from build123d import *

# Parameters (mm, degrees)
SKETCH1_W           = 50.8
SKETCH1_H           = 76.2
BOSS_EXTRUDE1_DEPTH = 1.6002
CUT_EXTRUDE1_REACH  = 47.818
SKETCH2_R           = 1.5875


with BuildPart() as part:
    # Sketch1 → Boss-Extrude1 (new body)
    with BuildSketch(Plane.XY):
        Rectangle(SKETCH1_W, SKETCH1_H)
    extrude(amount=BOSS_EXTRUDE1_DEPTH)

    # Sketch2 → Cut-Extrude1 (cut, up to next)
    with BuildSketch(Plane.XY.offset(1.6002), mode=Mode.PRIVATE) as cut_extrude1_sk1:
        with Locations((-21.59, 34.29)):
            Circle(SKETCH2_R)
    cut_extrude1_tool1 = extrude(cut_extrude1_sk1.sketch, amount=-CUT_EXTRUDE1_REACH, mode=Mode.PRIVATE) & part.part
    # Sketch2 → Cut-Extrude1 (cut, up to next)
    with BuildSketch(Plane.XY.offset(1.6002), mode=Mode.PRIVATE) as cut_extrude1_sk2:
        with Locations((21.59, 34.29)):
            Circle(SKETCH2_R)
    cut_extrude1_tool2 = extrude(cut_extrude1_sk2.sketch, amount=-CUT_EXTRUDE1_REACH, mode=Mode.PRIVATE) & part.part
    # Sketch2 → Cut-Extrude1 (cut, up to next)
    with BuildSketch(Plane.XY.offset(1.6002), mode=Mode.PRIVATE) as cut_extrude1_sk3:
        with Locations((21.59, -34.29)):
            Circle(SKETCH2_R)
    cut_extrude1_tool3 = extrude(cut_extrude1_sk3.sketch, amount=-CUT_EXTRUDE1_REACH, mode=Mode.PRIVATE) & part.part
    # Sketch2 → Cut-Extrude1 (cut, up to next)
    with BuildSketch(Plane.XY.offset(1.6002), mode=Mode.PRIVATE) as cut_extrude1_sk4:
        with Locations((-21.59, -34.29)):
            Circle(SKETCH2_R)
    cut_extrude1_tool4 = extrude(cut_extrude1_sk4.sketch, amount=-CUT_EXTRUDE1_REACH, mode=Mode.PRIVATE) & part.part
    add(cut_extrude1_tool1.solids().sort_by_distance((-21.59, 34.29, 1.6002))[0], mode=Mode.SUBTRACT)
    add(cut_extrude1_tool2.solids().sort_by_distance((21.59, 34.29, 1.6002))[0], mode=Mode.SUBTRACT)
    add(cut_extrude1_tool3.solids().sort_by_distance((21.59, -34.29, 1.6002))[0], mode=Mode.SUBTRACT)
    add(cut_extrude1_tool4.solids().sort_by_distance((-21.59, -34.29, 1.6002))[0], mode=Mode.SUBTRACT)


solid = part.part
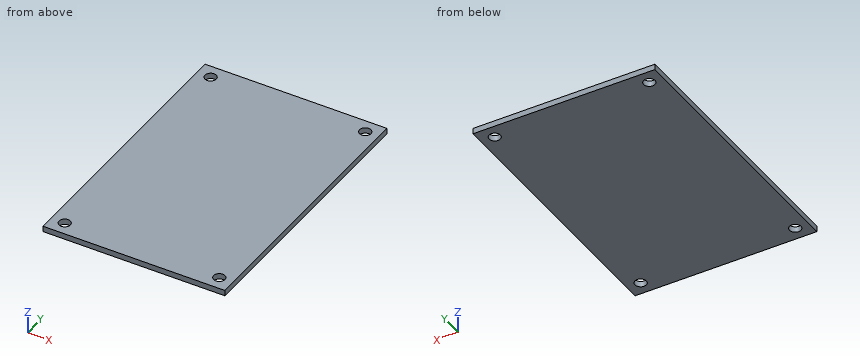
Input: part model. Units: mm. Frame: model coordinates. Coordinates: 2 decimals unless noted, no trailing zeros. Write each loop counter-clockwise with the first axis right and the second up, starting at its lowest first coordinate (ties: lowest second). Pieces come first, ordered by that corner, then holes. Notation, with made-up numbers: M 39,41 L 62,41 A16 cw 62,47 Z; hole C 46.25,47.5 d9. An arc over 180 degrees is marked long. Answer as a JSON object with one key per item and string values. Group by question number.
(1) Section B-B on x = 21.59. Output: boundary loops of the cut face in (y, z), plus the area to 3 significant figures.
(2) Ray query, line 1 along Y through (x, z) = (21.59, 1.2); line 2 along Y through (x, z) = (22, 1.2). Return the intervals inside material, ascending. Write a range as [from, to].
(3) Section A-A on y = 34.29. Output: boundary loops of the cut face in (x, z), plus the area to 3 significant figures.
Result set:
{
 "1": {"outline": "M -38.1,0 L -35.88,0 L -35.88,1.6 L -38.1,1.6 Z; M -32.7,0 L 32.7,0 L 32.7,1.6 L -32.7,1.6 Z; M 35.88,0 L 38.1,0 L 38.1,1.6 L 35.88,1.6 Z", "area": "112 mm2"},
 "2": {"line 1": "y = [-38.1, -35.88], [-32.7, 32.7], [35.88, 38.1]", "line 2": "y = [-38.1, -35.82], [-32.76, 32.76], [35.82, 38.1]"},
 "3": {"outline": "M -25.4,0 L -23.18,0 L -23.18,1.6 L -25.4,1.6 Z; M -20,0 L 20,0 L 20,1.6 L -20,1.6 Z; M 23.18,0 L 25.4,0 L 25.4,1.6 L 23.18,1.6 Z", "area": "71.1 mm2"}
}
